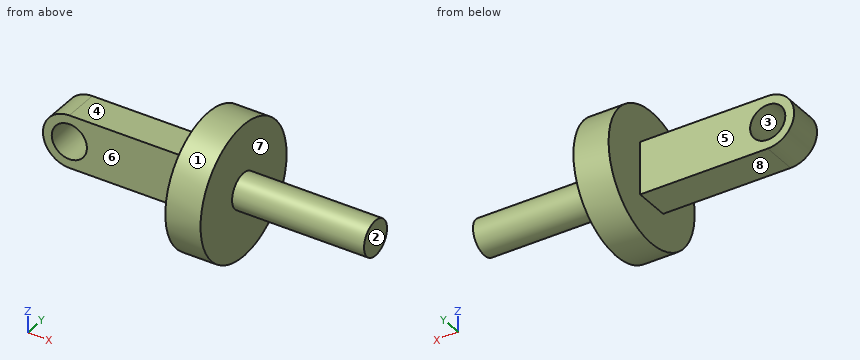
Autodesk Inventor part; units mm, degrees
ref_plane "YZ Plane" through (0, 0, 0) normal (1, 0, 0) x (0, 1, 0)
ref_plane "XZ Plane" through (0, 0, 0) normal (0, 1, 0) x (-1, 0, 0)
ref_plane "XY Plane" through (0, 0, 0) normal (0, 0, 1) x (1, 0, 0)
sketch "スケッチ1" plane through (0, 0, 0) normal (1, 0, 0) x (0, 1, 0)
  circle A0 centre (0, 0) radius 7.5
  dimension "d0" = 15
extrude "押し出し1" add sketch "スケッチ1" along normal blind 4
sketch "スケッチ2" plane through (0, 0, 0) normal (0, 1, 0) x (-1, 0, 0)
  circle A0 centre (14.5, 0) radius 2
  circle A1 centre (14.5, 0) radius 3
  line L0 (14.5, -3) -> (0, -3)
  line L1 (0, 7.5) -> (0, -7.5)
  line L2 (14.5, 3) -> (0, 3)
  point P0 (0, 0)
  dimension "d3" = 4
  dimension "d4" = 6
  dimension "d5" = 14.5
extrude "押し出し2" add sketch "スケッチ2" along normal mid plane 4
sketch "スケッチ3" plane through (4, 0, 0) normal (1, 0, 0) x (0, 0, -1)
  circle A0 centre (0, 0) radius 2
  dimension "d8" = 4
extrude "押し出し3" add sketch "スケッチ3" along normal blind 15
properties part number "black-suspension-top" material "ABS プラスチック"
Geometry check sheet. Reference: the model listing, model coordinates, mm. Face numbers are marked on the shaded views. A direction names the side the tool comes from. Round coordinates to 2 decimals unless told otherwise and drop trailing zeros. Order: outer loops, then holes, each group sorted by start corner. A loop starts at its lowest first (then second) coordinate and runs counter-clockwise, first axis right, second up. Notation, with made-up numbers: (15, -38) - (41, -38) arc R21 cw to (41, -17) - close; hole circle Ø7 at (3, 26.5). An arc over 180 degrees is marked (long way). Use a Markdown table: item, result. Add a question column.
(1) Sectioned sample at A-A, the plane z = 0. Enter the section's corners in (x, y).
(2) Depth check by flat-ended pin: pin 1 (4 mm diameter, centred on y = 2, z = 2, fed in from -X); pin 2 (6.5 mm diameter, centred on x = -14.5, z = 0, fed in from +Y); pin 3 (2 mm diameter, centred on x = 10.5, z = 2.5, fed in from +Y); pin 4 (2 mm diameter, centred on x = -12.5, y = 0.5, fed in from +Z). Enter the tip coordinate at first touch or a pass-through.
(3) Material ranges on line 1 along Z through (x, y) = (-14.5, 0.8); line 2 along X through (y, z) = (5.25, 1); line 3 along Y through (x, z) = (-8.5, 0.5), recorded low to high. Write a range as [from, to].
(4) Release check for a two-part mould opening along Z. For the marked faces 1, 2, 3 and 4 record: pulls with the +Z half, pulls with the -Z half, needs draft (parallel to the pull), parting line crosses it, or undercut.
(5) Sectioned sample at D-D, the plane y = 6. Enter the section's corners in (x, z), and give its area (3 significant figures).
(6) Sectioned sample at B-B, the plane y = 0. Enter the section's corners in (x, z), and give its area (3 significant figures).
(7) Sectioned sample at C-C, the plane x = 13.5. Enter the section's corners in (y, z), and give its area (3 significant figures).
(8) Tool access check on the marked faces 5, 6, 7 and 8. Record the directions out of +Z, -Z, +X, -X, +Y, -Y that give a thin tool (end or side, any length) a straight path to the whole face; none if there is none.
Answers below:
| question | item | result |
|---|---|---|
| 1 | outline | (-17.5, -2) - (-16.5, -2) - (-16.5, 2) - (-17.5, 2) - close; (-12.5, -2) - (0, -2) - (0, -7.5) - (4, -7.5) - (4, -2) - (19, -2) - (19, 2) - (4, 2) - (4, 7.5) - (0, 7.5) - (0, 2) - (-12.5, 2) - close |
| 2 | pin 1 | x = -17.5 |
| 2 | pin 2 | y = 2 |
| 2 | pin 3 | y = 1.32 |
| 2 | pin 4 | z = 3 |
| 3 | line 1 | [-3, -2], [2, 3] |
| 3 | line 2 | [0, 4] |
| 3 | line 3 | [-2, 2] |
| 4 | face 1 | parting line crosses it |
| 4 | face 2 | needs draft |
| 4 | face 3 | undercut |
| 4 | face 4 | pulls with the +Z half |
| 5 | outline | (0, -4.5) - (4, -4.5) - (4, 4.5) - (0, 4.5) - close |
| 5 | area | 36.0 mm² |
| 6 | outline | (-14.5, -3) - (0, -3) - (0, -7.5) - (4, -7.5) - (4, -2) - (19, -2) - (19, 2) - (4, 2) - (4, 7.5) - (0, 7.5) - (0, 3) - (-14.5, 3) arc R3 ccw to start; hole circle Ø4 at (-14.5, 0) |
| 6 | area | 209 mm² |
| 7 | outline | circle Ø4 at (0, 0) |
| 7 | area | 12.6 mm² |
| 8 | face 5 | +Z, -Z, -X, +Y |
| 8 | face 6 | +Z, -Z, -X, -Y |
| 8 | face 7 | +X |
| 8 | face 8 | -Z, -X, +Y, -Y |
